Part print with two shaded views. Sizes in mm from the minimum x, y, z corner. A direction names the side the tool comes from. Give positions to 0.01 mm unless a question says otherwise; leave off trailing zeros. Write each loop counter-clockwise with the first axis right and the second up, starting at its lowest first coordinate (ties: lowest second). Pieces come first, ordered by that corner, then holes. Notation, with made-up numbers: (40, 5.25) -> (70, 5.25) arc R30 cw to (70, 29.25) -> close; hole circle Ø2 at (-19, -7). An arc over 180 degrees is marked (long way). Answer as a JSON object with one key per item and string values.
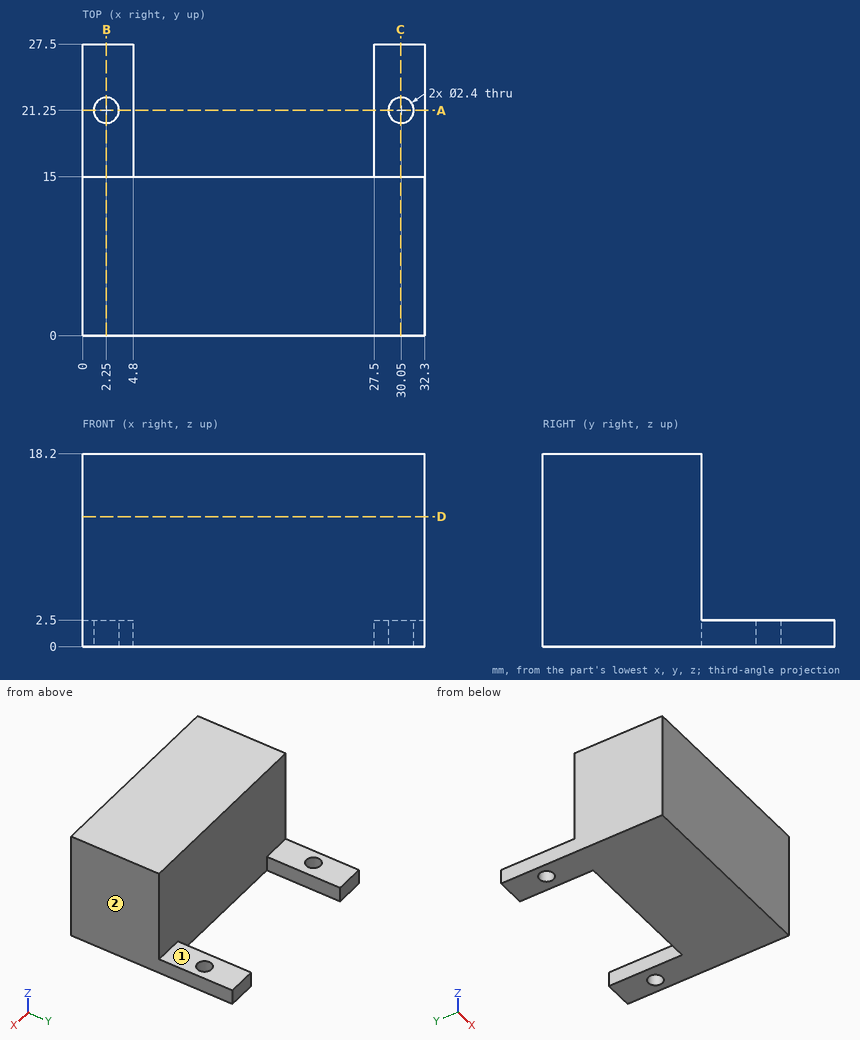
1) Slice it at A-A (y = 21.25). List the corners of the cut face in (x, z).
Model answer:
{"outline": "(0, 0) -> (1.05, 0) -> (1.05, 2.5) -> (0, 2.5) -> close; (3.45, 0) -> (4.8, 0) -> (4.8, 2.5) -> (3.45, 2.5) -> close; (27.5, 0) -> (28.85, 0) -> (28.85, 2.5) -> (27.5, 2.5) -> close; (31.25, 0) -> (32.3, 0) -> (32.3, 2.5) -> (31.25, 2.5) -> close"}
2) Slice it at D-D (z = 12.25). List the corners of the cut face in (x, y).
Model answer:
{"outline": "(0, 0) -> (32.3, 0) -> (32.3, 15) -> (0, 15) -> close"}
3) Wall check: probe 1 along Y at (x, z) = (30.05, 0.5); probe 2 along Y at (x, z) = (3.5, 10.5); probe 3 along Z at (x, y) = (30, 16.25). Give the ranges that are in metal, low to high.
Model answer:
{"probe 1": "y = 0 to 20.05, 22.45 to 27.5", "probe 2": "y = 0 to 15", "probe 3": "z = 0 to 2.5"}
4) 3-axis set-ups, long thin cutter, end or side, ignore diameter. For the marked faces 1 and 2: which of +Z, -Z, +X, -X, +Y, -Y reach the whole face in a straight line?
Model answer:
{"face 1": "+Z, +X, -X, +Y", "face 2": "+Z, -Z, +X, +Y, -Y"}
5) Slice it at B-B (x = 2.25). List the corners of the cut face in (y, z), then the cut area to 3 significant figures.
Model answer:
{"outline": "(0, 0) -> (20.05, 0) -> (20.05, 2.5) -> (15, 2.5) -> (15, 18.2) -> (0, 18.2) -> close; (22.45, 0) -> (27.5, 0) -> (27.5, 2.5) -> (22.45, 2.5) -> close", "area": "298 mm2"}
6) Pin check, flat tips, straight feed: pin 1 (4 mm diameter, centred on x = 29, y = 23, fed in from +Z); pin 2 (3 mm diameter, centred on y = 19, z = 1, fed in from -X); pin 3 (1.5 mm diameter, centred on x = 14, z = 10, fed in from +Y). Stop position of each tip, or through.
Model answer:
{"pin 1": "stops at z = 2.5", "pin 2": "stops at x = 0", "pin 3": "stops at y = 15"}
